```python
from build123d import *

# Parameters (mm, degrees)
SKETCH1_R             = 4
BASE_EXTRUDE_DEPTH    = 3.6
RBODY_SKETCH_R        = 5.55
RBODY_DEPTH           = 9.3
ELBOW_ANGLE           = 90
SKETCH3_R             = 4
BOSS_EXTRUDE1_DEPTH   = 9.8
NUT_DEPTH             = 4.59
THREAD_CHAMFER_SIZE   = 0.25
RTUBE_START           = -13.3
RTUBE_SKETCH_R        = 3.175
RTUBE_DEPTH           = 13.3
RTUBE_RADIUS_R        = 0.5
DIAMETER_R            = 2.25
PORT_THREADS_REACH    = 31.53
PORT_THREADS_SKETCH_R = 2.25


with BuildPart() as part:
    # Sketch1 → Base-Extrude (new body)
    with BuildSketch(Plane(origin=(0, 0, 0), x_dir=(0, 0, -1), z_dir=(1, 0, 0))):
        with Locations(Location((0, 0, 0), (0, 0, 180))):
            Circle(SKETCH1_R)
    extrude(amount=BASE_EXTRUDE_DEPTH)

    # RBody_Sketch → RBody (add)
    with BuildSketch(Plane(origin=(3.6, 0, 0), x_dir=(0, 0, -1), z_dir=(1, 0, 0))):
        with Locations(Location((0, 0, 0), (0, 0, 180))):
            Circle(RBODY_SKETCH_R)
    extrude(amount=RBODY_DEPTH)

    # RBody_Chamfer: read off the stored shape, not the designer's step
    # RBody_Chamfer outline → RBody_Chamfer (revolve, cut)
    with BuildSketch(Plane.YX):
        Polygon((5.55, 4.164153863), (4, 3.6), (5.55, 3.6), align=None)
    revolve(axis=Axis((0, 0, 0), (1, 0, 0)), mode=Mode.SUBTRACT)

    # RRelease_Sketch → RRelease (revolve)
    with BuildSketch(Plane.XY, mode=Mode.PRIVATE) as rrelease_sk:
        with BuildLine():
            Line((12.9, 3.575), (14.1, 3.575))
            Line((14.1, 3.575), (14.1, 5.025))
            Line((14.1, 5.025), (15.1, 5.025))
            ThreePointArc((15.1, 5.025), (15.453553391, 4.878553391), (15.6, 4.525))
            Line((15.6, 4.525), (15.6, 0))
            Line((15.6, 0), (12.9, 0))
            Line((12.9, 0), (12.9, 3.575))
        make_face()
    revolve(rrelease_sk.sketch.rotate(Axis((12.597722381, 0, 0), (1, 0, 0)), 90), axis=Axis((12.597722381, 0, 0), (1, 0, 0)))

    # Elbow_Sketch → Elbow (revolve)
    with BuildSketch(Plane.ZY):
        with BuildLine():
            Line((-4, 0), (4, 0))
            ThreePointArc((4, 0), (0, 4), (-4, 0))
        make_face()
    revolve(axis=Axis((0, 0, -6.487672297), (0, 0, 1)), revolution_arc=ELBOW_ANGLE)

    # Sketch3 → Boss-Extrude1 (add)
    with BuildSketch(Plane.XZ):
        with Locations(Location((0, 0, 0), (0, 0, 90))):
            Circle(SKETCH3_R)
    extrude(amount=BOSS_EXTRUDE1_DEPTH)

    # Nut_Sketch → Nut (add)
    with BuildSketch(Plane(origin=(0, -14.39, 0), x_dir=(-1, 0, 0), z_dir=(0, 1, 0))):
        Polygon((6.414361491, 0), (3.207180745, 5.555), (-3.207180745, 5.555), (-6.414361491, 0), (-3.207180745, -5.555), (3.207180745, -5.555), align=None)
    extrude(amount=NUT_DEPTH)

    # Nut_Chamfer_Sketch → Nut_Chamfer (revolve, cut)
    with BuildSketch(Plane.XY):
        Polygon((-5.555, -9.8), (-6.414361491, -9.8), (-6.414361491, -10.296152588), align=None)
        Polygon((-6.414361491, -13.893847412), (-5.555, -14.39), (-6.414361491, -14.39), align=None)
    revolve(axis=Axis((0, -1.551633987, 0), (0, 1, 0)), mode=Mode.SUBTRACT)

    # Thread_Sketch → Thread (revolve)
    with BuildSketch(Plane.XY):
        Polygon((0, -14.39), (-4.325, -14.39), (-4.325, -15.35), (-4.864, -15.35), (-4.864, -18.9), (0, -18.9), align=None)
    revolve(axis=Axis((0, 0, 0), (0, -1, 0)))

    # Thread_Chamfer
    thread_chamfer_edges = [part.edges().sort_by_distance(p)[0] for p in [
        (4.864, -18.9, 0),
        (4.864, -15.35, 0),
    ]]
    chamfer(thread_chamfer_edges, length=THREAD_CHAMFER_SIZE)

    # Sketch6 → Cut-Revolve1 (revolve, cut)
    with BuildSketch(Plane.XY):
        Polygon((-4.325, -14.39), (-6.414361491, -14.39), (-6.414361491, -12.300638509), align=None)
    revolve(axis=Axis((0, -7.772283854, 0), (0, -1, 0)), mode=Mode.SUBTRACT)

    # RTube_Sketch → RTube (cut)
    with BuildSketch(Plane(origin=(15.6, 0, 0), x_dir=(0, 0, -1), z_dir=(1, 0, 0)).offset(RTUBE_START)):
        Circle(RTUBE_SKETCH_R)
    extrude(amount=RTUBE_DEPTH, mode=Mode.SUBTRACT)

    # RTube_Radius
    rtube_radius_edges = [part.edges().sort_by_distance(p)[0] for p in [
        (15.6, 0, 3.175),
    ]]
    fillet(rtube_radius_edges, radius=RTUBE_RADIUS_R)

    # Port_Curve: sweep along a path in Profile
    with BuildLine(Plane.XY) as port_curve_path:
        ThreePointArc((2.3, 0), (0.673654403, -0.673654403), (0, -2.3))
    # Diameter → Port_Curve (sweep, cut)
    with BuildSketch(Plane(origin=(2.3, 0, 0), x_dir=(0, 0, -1), z_dir=(1, 0, 0))):
        Circle(DIAMETER_R)
    sweep(path=port_curve_path.line, mode=Mode.SUBTRACT)

    # Port_Threads_Sketch → Port_Threads (cut, up to next)
    with BuildSketch(Plane(origin=(0, -18.9, 0), x_dir=(-1, 0, 0), z_dir=(0, 1, 0)), mode=Mode.PRIVATE) as port_threads_sk1:
        Circle(PORT_THREADS_SKETCH_R)
    port_threads_tool1 = extrude(port_threads_sk1.sketch, amount=PORT_THREADS_REACH, mode=Mode.PRIVATE) & part.part
    add(port_threads_tool1.solids().sort_by_distance((0, -18.9, 0))[0], mode=Mode.SUBTRACT)


solid = part.part
```
The model under review builds one solid part; all positions refer to its coordinate system, in mm. A direction names the side the tool comes from. Round coordinates to 2 decimals unless told otherwise and drop trailing zeros. Order: outer loops, then holes, each group sorted by start corner. A loop starts at its lowest first (then second) coordinate and runs counter-clockwise, first axis right, second up.
(1) Take a section at C-C, the plane x = 6. Count the separate pieces of the cut face and the enclosed holes in it, plus the area to 3 significant figures.
Working result:
separate pieces: 2
enclosed holes: 1
area: 68.9 mm2
(2) Take a section at B-B, the plane y = -15. State the section outline as (x, z) points (3 decimals), plus the area to 3 significant figures.
Working result:
outline: circle Ø8.65 at (0, 0); hole circle Ø4.5 at (0, 0)
area: 42.9 mm2
(3) For P1, Ø2, axis at x = 0, z = 3, coming from the +Y side; P2, Ø3, axis at y = 1.5, z = 0.5, coming from the +X side; P3, Ø3, axis at y = -1.5, z = 2.5, coming from the -X side, all flat-tipped, find the tip position at first contact; note any pin that passes through.
Working result:
P1: stops at y = 3.46
P2: stops at x = 2.3
P3: stops at x = -3.87
(4) Take a section at A-A, the plane x = 10.25. State the section outline as (y, z) points (3 decimals).
Working result:
outline: circle Ø11.1 at (0, 0); hole circle Ø6.35 at (0, 0)
(5) Tool access review of faces 5 (the face through (2.892, -9.918, -4.981)), 6 (the face through (13.508, -3.545, -0.465)), 7 (the face through (2.3, -2.1, -1.4)): name each direction out of +Z, -Z, +X, -X, +Y, -Y from which nothing blocks a thin tool from reaching the whole face with its end or side.
Working result:
face 5: -Z, +X
face 6: none
face 7: +X
(6) Wall thickness on L1, parallel to Y at x = 5.75, z = 0.25; L2, parallel to Y at x = 4.75, z = 0.5; L3, parallel to Y at x = 13, z = 2.5: over which ranges is each line inside the solid? List them lowest first.
Working result:
L1: y = -12.96 to -9.92, -5.54 to -3.17, 3.17 to 5.54
L2: y = -18.74 to -15.51, -13.94 to -9.8, -5.53 to -3.14, 3.14 to 5.53
L3: y = -2.56 to -1.96, 1.96 to 2.56
(7) Mouldability with a two-part tool opening along X and no side actions: class faces 1 (the face through (8.61, -3.1, 0.69)), 2 (the face through (3.69, 4.05, 1.28)), 3 (the face through (-5.76, -9.92, -0.01)), 4 (the face through (4.833, -11.504, -2.739)) as released by +X, released by -X, zero draft, split by the parting line, or undercut.
Working result:
face 1: zero draft
face 2: undercut
face 3: released by -X
face 4: released by +X
